Geometry: final body of the model. Coordinates: model frame, mm. A direction names the side the tool comes from. Coordinates: 2 decimals unless noted, no trailing zeros. Order: outer loops, then holes, each group sorted by start corner. A loop starts at its lowest first (then second) coordinate and runs counter-clockwise, first axis right, second up. Notation, with made-up numbers: M -1,-21 L 5,-21 A17 cw 5,-8 Z; hole C -25.75,46.25 d10. An arc over 180 degrees is marked long. Use CSV: the item, a comma, the result in double quotes. Start each with the question number.
Q1. Access query for faces 5 (the face through (27.554, -0.217, -0.976)), 6 (the face through (28.05, -1.5, 0.07)), 7 (the face through (10, 0, -2)). Directions: +Z, -Z, +X, -X, +Y, -Y. A direction counts if a zero-diameter tool reaches every point of the face in a straight line with its end or side. Return the directions, or none.
Q2. Section query B-B, the plane x = 16. Output: boundary loops of the cut face in (y, z), and give its area (3 significant figures).
Q3. Ray query, probe 1 along Y at (x, z) = (3.7, 0); probe 2 along Y at (x, z) = (18, 0.15). Return the intervals inside material, ascending.
Q4. First-contact query: P1, Ø1, axis at x = 5, z = -1, coming from the -Y side; P2, Ø1, axis at y = -0.5, z = 0.5, coming from the -X side; P3, Ø1.5, axis at y = 0.5, z = -0.5, coming from the -X side. Flat tips, straight axial feed; report the tip coordinate or a pass-through.
Q5. Section query A-A, the plane x = 2.75. Output: boundary loops of the cut face in (y, z), and give its area (3 significant figures).
Q6. Mould query, pull axis Z, two halves, no side actions, for faces 1 (the face through (6.745, -0.254, -0.056)), 2 (the face through (28.3, 0, 0)), 3 (the face through (3.04, -0.07, -1.5)), 4 (the face through (23.8, -1.5, 0.07)). Classes: +Z half, -Z half, draft (parallel to the pull), parting line (faces both ways), or undercut.
Autodesk Inventor part; units mm, degrees
ref_plane "YZ Plane" through (0, 0, 0) normal (1, 0, 0) x (0, 1, 0)
ref_plane "XZ Plane" through (0, 0, 0) normal (0, 1, 0) x (-1, 0, 0)
ref_plane "XY Plane" through (0, 0, 0) normal (0, 0, 1) x (1, 0, 0)
sketch "Sketch1" plane through (0, 0, 0) normal (0, 0, 1) x (1, 0, 0)
  line L0 (0, 0) -> (0, 2)
  line L1 (0, 2) -> (20.2, 2)
  line L2 (20.2, 2) -> (20.2, 1.5)
  line L3 (20.2, 1.5) -> (27.3, 1.5)
  line L4 (27.3, 1.5) -> (27.3, 1)
  line L5 (27.3, 1) -> (27.8, 1)
  line L6 (27.8, 1) -> (27.8, 1.5)
  line L7 (27.8, 1.5) -> (28.3, 1.5)
  line L8 (28.3, 1.5) -> (28.3, 0)
  line L9 (28.3, 0) -> (0, 0)
  dimension "d0" = 4
  dimension "d1" = 3
  dimension "d2" = 0.5
  dimension "d3" = 0.5
  dimension "d4" = 0.5
  dimension "d5" = 7.1
  dimension "d6" = 20.2
revolve "Revolution1" add sketch "Sketch1" angle 360 about axis through (28.3, 0, 0) along (-1, 0, 0)
hole "Hole1" at (0, 0, 0) direction (1, 0, 0) diameter 3 depth 6 tip angle 118
properties part number "thumb_opposing_worm_shaft" material "Stainless Steel"
Responses:
1,face 5,"none"
1,face 6,"+X"
1,face 7,"+X, -X"
2,outline,"C 0,0 d4"
2,area,"12.6 mm²"
3,probe 1,"y = -2 to -1.5, 1.5 to 2"
3,probe 2,"y = -1.99 to 1.99"
4,P1,"stops at y = -1.94"
4,P2,"stops at x = 6.18"
4,P3,"stops at x = 6.03"
5,outline,"C 0,0 d4; hole C 0,0 d3"
5,area,"5.50 mm²"
6,face 1,"undercut"
6,face 2,"draft"
6,face 3,"undercut"
6,face 4,"parting line"
